```python
from build123d import *

# Parameters (mm, degrees)
EXTRUDE_1_DEPTH     = 6
EXTRUDE_2_DEPTH     = 12
CUT_EXTRUDE_1_REACH = 52.712
SKETCH_3_R          = 1.5
CHAMFER_1_SIZE      = 2
SKETCH_4_W          = 27
SKETCH_4_H          = 48.5
EXTRUDE_3_DEPTH     = 6.9
SKETCH_5_W          = 32.5
SKETCH_5_H          = 0.5
CUT_EXTRUDE_2_DEPTH = 51.711956184
SKETCH_6_W          = 5
SKETCH_6_H          = 5
EXTRUDE_4_DEPTH     = 6
SKETCH_9_R          = 1.25
CUT_EXTRUDE_5_DEPTH = 54.113110434
SKETCH_10_R         = 2
CUT_EXTRUDE_6_DEPTH = 4
CHAMFER_3_SIZE      = 3.5


with BuildPart() as part:
    # 草图1 → 凸台-拉伸1 (new body)
    with BuildSketch(Plane(origin=(0, 0, 0), x_dir=(1, 0, 0), z_dir=(0, 1, 0))):
        Polygon((-25.45, -32), (-25.45, -28), (-25.45, -3.5), (-25.45, 0.5), (-25.45, 8.5), (-16.25, 8.5), (-16.25, 38.5), (16.25, 38.5), (16.25, 8.5), (25.45, 8.5), (25.45, 0.5), (25.45, -3.5), (25.45, -28), (25.45, -32), (25.45, -40), (-25.45, -40), align=None)
    extrude(amount=EXTRUDE_1_DEPTH)

    # 草图2 → 凸台-拉伸2 (add)
    with BuildSketch(Plane(origin=(0, 6, 0), x_dir=(1, 0, 0), z_dir=(0, 1, 0))):
        Polygon((-4, 22.9), (-4, 8.5), (4, 8.5), (4, 22.9), (9.2, 22.9), (9.2, 38.5), (-9.2, 38.5), (-9.2, 22.9), align=None)
    extrude(amount=EXTRUDE_2_DEPTH)

    # 草图3 → 切除-拉伸1 (cut, up to next)
    with BuildSketch(Plane.XZ, mode=Mode.PRIVATE) as cut_extrude_1_sk1:
        with Locations(Location((13.25, -32.5, 0), (0, 0, 270))):
            Circle(SKETCH_3_R)
    cut_extrude_1_tool1 = extrude(cut_extrude_1_sk1.sketch, amount=-CUT_EXTRUDE_1_REACH, mode=Mode.PRIVATE) & part.part
    # 草图3 → 切除-拉伸1 (cut, up to next)
    with BuildSketch(Plane.XZ, mode=Mode.PRIVATE) as cut_extrude_1_sk2:
        with Locations(Location((10.25, -15, 0), (0, 0, 270))):
            Circle(SKETCH_3_R)
    cut_extrude_1_tool2 = extrude(cut_extrude_1_sk2.sketch, amount=-CUT_EXTRUDE_1_REACH, mode=Mode.PRIVATE) & part.part
    # 草图3 → 切除-拉伸1 (cut, up to next)
    with BuildSketch(Plane.XZ, mode=Mode.PRIVATE) as cut_extrude_1_sk3:
        with Locations(Location((-13.25, -32.5, 0), (0, 0, 90))):
            Circle(SKETCH_3_R)
    cut_extrude_1_tool3 = extrude(cut_extrude_1_sk3.sketch, amount=-CUT_EXTRUDE_1_REACH, mode=Mode.PRIVATE) & part.part
    # 草图3 → 切除-拉伸1 (cut, up to next)
    with BuildSketch(Plane.XZ, mode=Mode.PRIVATE) as cut_extrude_1_sk4:
        with Locations(Location((-10.25, -15, 0), (0, 0, 90))):
            Circle(SKETCH_3_R)
    cut_extrude_1_tool4 = extrude(cut_extrude_1_sk4.sketch, amount=-CUT_EXTRUDE_1_REACH, mode=Mode.PRIVATE) & part.part
    # 草图3 → 切除-拉伸1 (cut, up to next)
    with BuildSketch(Plane.XZ, mode=Mode.PRIVATE) as cut_extrude_1_sk5:
        with BuildLine():
            Line((13.5, 19), (13.5, 35))
            ThreePointArc((13.5, 35), (17, 38.5), (20.5, 35))
            Line((20.5, 35), (20.5, 19))
            ThreePointArc((20.5, 19), (17, 15.5), (13.5, 19))
        make_face()
    cut_extrude_1_tool5 = extrude(cut_extrude_1_sk5.sketch, amount=-CUT_EXTRUDE_1_REACH, mode=Mode.PRIVATE) & part.part
    # 草图3 → 切除-拉伸1 (cut, up to next)
    with BuildSketch(Plane.XZ, mode=Mode.PRIVATE) as cut_extrude_1_sk6:
        with BuildLine():
            Line((-13.5, 19), (-13.5, 35))
            ThreePointArc((-13.5, 35), (-17, 38.5), (-20.5, 35))
            Line((-20.5, 35), (-20.5, 19))
            ThreePointArc((-20.5, 19), (-17, 15.5), (-13.5, 19))
        make_face()
    cut_extrude_1_tool6 = extrude(cut_extrude_1_sk6.sketch, amount=-CUT_EXTRUDE_1_REACH, mode=Mode.PRIVATE) & part.part
    add(cut_extrude_1_tool1.solids().sort_by_distance((13.25, 0, -32.5))[0], mode=Mode.SUBTRACT)
    add(cut_extrude_1_tool2.solids().sort_by_distance((10.25, 0, -15))[0], mode=Mode.SUBTRACT)
    add(cut_extrude_1_tool3.solids().sort_by_distance((-13.25, 0, -32.5))[0], mode=Mode.SUBTRACT)
    add(cut_extrude_1_tool4.solids().sort_by_distance((-10.25, 0, -15))[0], mode=Mode.SUBTRACT)
    add(cut_extrude_1_tool5.solids().sort_by_distance((17, 0, 27))[0], mode=Mode.SUBTRACT)
    add(cut_extrude_1_tool6.solids().sort_by_distance((-17, 0, 27))[0], mode=Mode.SUBTRACT)

    # 倒角1
    chamfer_1_edges = [part.edges().sort_by_distance(p)[0] for p in [
        (0, 18, -8.5),
    ]]
    chamfer(chamfer_1_edges, length=CHAMFER_1_SIZE)

    # 草图4 → 凸台-拉伸3 (add)
    with BuildSketch(Plane(origin=(0, 6, 0), x_dir=(1, 0, 0), z_dir=(0, 1, 0))):
        with Locations((0, -15.75)):
            Rectangle(SKETCH_4_W, SKETCH_4_H)
    extrude(amount=EXTRUDE_3_DEPTH)

    # 草图5 → 切除-拉伸2 (cut, through all)
    with BuildSketch(Plane.XZ):
        Polygon((24.95, 40), (24.95, -8), (16.25, -8), (16.25, -8.5), (25.45, -8.5), (25.45, 40), align=None)
        Polygon((-16.25, -8.5), (-25.45, -8.5), (-25.45, 40), (-24.95, 40), (-24.95, -8), (-16.25, -8), align=None)
        with Locations((0, -38.25)):
            Rectangle(SKETCH_5_W, SKETCH_5_H)
    extrude(amount=-CUT_EXTRUDE_2_DEPTH, mode=Mode.SUBTRACT)

    # 草图6 → 凸台-拉伸4 (add)
    with BuildSketch(Plane.XZ):
        with Locations((-27.45, 29)):
            Rectangle(SKETCH_6_W, SKETCH_6_H)
        with Locations((27.45, 29)):
            Rectangle(SKETCH_6_W, SKETCH_6_H)
    extrude(amount=-EXTRUDE_4_DEPTH)

    # 草图9 → 切除-拉伸5 (cut, through all)
    with BuildSketch(Plane.XZ):
        with Locations(Location((-27.7, 29, 0), (0, 0, 270))):
            Circle(SKETCH_9_R)
        with Locations(Location((27.7, 29, 0), (0, 0, 270))):
            Circle(SKETCH_9_R)
    extrude(amount=-CUT_EXTRUDE_5_DEPTH, mode=Mode.SUBTRACT)

    # 草图10 → 切除-拉伸6 (cut)
    with BuildSketch(Plane.XZ):
        with Locations(Location((27.7, 29, 0), (0, 0, 270))):
            Circle(SKETCH_10_R)
        with Locations(Location((-27.7, 29, 0), (0, 0, 270))):
            Circle(SKETCH_10_R)
    extrude(amount=-CUT_EXTRUDE_6_DEPTH, mode=Mode.SUBTRACT)

    # 倒角3
    # the kernel refuses this chamfer: 3.5 mm, written as the material it takes off along each edge
    with BuildSketch(Plane(origin=(10.25, 0, -15), x_dir=(0, 0, -1), z_dir=(-1, 0, 0))) as chamfer_3_piece_1:
        Polygon((1.5 + CHAMFER_3_SIZE, 0), (1.5, -CHAMFER_3_SIZE), (1.5, 0), align=None)
    revolve(axis=Axis((10.25, 0, -15), (0, -1, 0)), mode=Mode.SUBTRACT)
    with BuildSketch(Plane(origin=(-13.25, 0, -32.5), x_dir=(0, 0, 1), z_dir=(1, 0, 0))) as chamfer_3_piece_2:
        Polygon((1.5, -CHAMFER_3_SIZE), (1.5 + CHAMFER_3_SIZE, 0), (1.5, 0), align=None)
    revolve(axis=Axis((-13.25, 0, -32.5), (0, -1, 0)), mode=Mode.SUBTRACT)
    with BuildSketch(Plane(origin=(13.25, 0, -32.5), x_dir=(0, 0, -1), z_dir=(-1, 0, 0))) as chamfer_3_piece_3:
        Polygon((1.5 + CHAMFER_3_SIZE, 0), (1.5, -CHAMFER_3_SIZE), (1.5, 0), align=None)
    revolve(axis=Axis((13.25, 0, -32.5), (0, -1, 0)), mode=Mode.SUBTRACT)
    with BuildSketch(Plane(origin=(-10.25, 0, -15), x_dir=(0, 0, 1), z_dir=(1, 0, 0))) as chamfer_3_piece_4:
        Polygon((1.5, -CHAMFER_3_SIZE), (1.5 + CHAMFER_3_SIZE, 0), (1.5, 0), align=None)
    revolve(axis=Axis((-10.25, 0, -15), (0, -1, 0)), mode=Mode.SUBTRACT)


solid = part.part
```
Work out the finished part from the listing and answer in its coordinate system (mm). A direction names the side the tool comes from. Give positions to 0.01 mm unless a question says otherwise; leave off trailing zeros. Order: outer loops, then holes, each group sorted by start corner. A loop starts at its lowest first (then second) coordinate and runs counter-clockwise, first axis right, second up.
1. The mould has two halves that part along X. Classify faces 1 (the flat face through (-4, 12, -16)), 2 (the cylindrical face through (-17.1, 3, 15.5)), 3 (the flat face through (24.95, 3, 36)): released by +X, released by -X, zero draft, split by the parting line, or undercut.
Result sheet:
face 1: released by -X
face 2: undercut
face 3: released by +X
2. Section C-C, the plane z = -15 is taken. Determine the outline of the cut face in (x, y).
Result sheet:
outline: (-16.25, 0) - (-15.25, 0) - (-11.75, 3.5) - (-11.75, 6) - (-16.25, 6) - close; (-8.75, 3.5) - (-5.25, 0) - (5.25, 0) - (8.75, 3.5) - (8.75, 6) - (4, 6) - (4, 18) - (-4, 18) - (-4, 6) - (-8.75, 6) - close; (11.75, 3.5) - (15.25, 0) - (16.25, 0) - (16.25, 6) - (11.75, 6) - close
3. Straight lines are drawn through the part: L1, parallel to X at y = 1, z = 36.5; L2, parallel to X at y = 11.75, z = -4.5; L3, parallel to Y at x = 9.5, z = 31.5. For each, find the intervals that lie inside material, in ascending order.
Result sheet:
L1: x = -24.95 to -20.16, -13.84 to 13.84, 20.16 to 24.95
L2: x = -13.5 to 13.5
L3: y = 0 to 12.9
4. Each of these flat-tipped pins is pushed along its axis until it touches: P1, Ø0.9, axis at x = 2, y = 15, coming from the +Z side; P2, Ø3, axis at y = 2.5, z = 24.5, coming from the -X side; P3, Ø4, axis at x = 28, y = 3.5, coming from the +Z side. Where does it stop, or does it pass through?
Result sheet:
P1: stops at z = -8.5
P2: stops at x = -24.95
P3: stops at z = 31.5
5. For faces 4 (the cylindrical face through (17.1, 3, 15.5)), 5 (the flat face through (-7, 12, -22.9)), 6 (the flat face through (-16.25, 3, -23)), determine the directions among +Z, -Z, +X, -X, +Y, -Y from which every point of the face is accessible in a straight line to the end or side of a thin tool.
Result sheet:
face 4: +Y, -Y
face 5: -X, +Y
face 6: -Z, -X, +Y, -Y
6. Section B-B, the plane y = 1.75 is taken. Give the number of separate pieces and of enclosed holes in the cut face, and give its area (3 significant figures).
Result sheet:
separate pieces: 1
enclosed holes: 6
area: 2,960 mm2
7. Section A-A, the plane z = 29 is taken. Determine the outline of the cut face in (x, y).
Result sheet:
outline: (-29.95, 0) - (-29.7, 0) - (-29.7, 4) - (-28.95, 4) - (-28.95, 6) - (-29.95, 6) - close; (-26.45, 4) - (-25.7, 4) - (-25.7, 0) - (-20.5, 0) - (-20.5, 6) - (-26.45, 6) - close; (-13.5, 0) - (13.5, 0) - (13.5, 12.9) - (-13.5, 12.9) - close; (20.5, 0) - (25.7, 0) - (25.7, 4) - (26.45, 4) - (26.45, 6) - (20.5, 6) - close; (28.95, 4) - (29.7, 4) - (29.7, 0) - (29.95, 0) - (29.95, 6) - (28.95, 6) - close
8. Section D-D, the plane x = 19 is taken. Determine the outline of the cut face in (y, z).
Result sheet:
outline: (0, -8) - (6, -8) - (6, 16.13) - (0, 16.13) - close; (0, 37.87) - (6, 37.87) - (6, 40) - (0, 40) - close
